from build123d import *

# Parameters (mm, degrees)
MODEL_W                         = 27.94
MODEL_H                         = 50.8
MODEL_R                         = 1.05
MODEL_R_2                       = 5.08
BOSS_EXTRUDE1_DEPTH             = 3.175
F_43_0_089_DIAMETER_HOLE1_D     = 2.2606
F_43_0_089_DIAMETER_HOLE1_DEPTH = 25.4
F_43_0_089_DIAMETER_HOLE1_TIP   = 0.679152758


with BuildPart() as part:
    # Model → Boss-Extrude1 (new body)
    with BuildSketch(Plane.XY):
        with Locations((0, 11.43)):
            Rectangle(MODEL_W, MODEL_H)
        with Locations((-6.92820323, 4.000000001)):
            Circle(MODEL_R, mode=Mode.SUBTRACT)
        with Locations((-6.92820323, -4.000000001)):
            Circle(MODEL_R, mode=Mode.SUBTRACT)
        with Locations((0, -7.999999999)):
            Circle(MODEL_R, mode=Mode.SUBTRACT)
        with Locations((6.92820323, -4.000000001)):
            Circle(MODEL_R, mode=Mode.SUBTRACT)
        with Locations((6.92820323, 4.000000001)):
            Circle(MODEL_R, mode=Mode.SUBTRACT)
        with Locations((0, 7.999999999)):
            Circle(MODEL_R, mode=Mode.SUBTRACT)
        Circle(MODEL_R_2, mode=Mode.SUBTRACT)
    extrude(amount=BOSS_EXTRUDE1_DEPTH)

    # #43 (0.089) Diameter Hole1
    with Locations(Plane.XY.offset(3.175)):
        with Locations((-7.39143302, 7.395974597)):
            Hole(F_43_0_089_DIAMETER_HOLE1_D / 2, depth=F_43_0_089_DIAMETER_HOLE1_DEPTH)
            with Locations((0, 0, -(F_43_0_089_DIAMETER_HOLE1_DEPTH + F_43_0_089_DIAMETER_HOLE1_TIP / 2))):  # 118° drill point
                Cone(0, F_43_0_089_DIAMETER_HOLE1_D / 2, F_43_0_089_DIAMETER_HOLE1_TIP, mode=Mode.SUBTRACT)


solid = part.part
Build history of the part. All positions in model axes, mm. Give positions to 0.01 mm unless a question says otherwise; leave off trailing zeros. Order: outer loops, then holes, each group sorted by start corner. A loop starts at its lowest first (then second) coordinate and runs counter-clockwise, first axis right, second up. Notation, with made-up numbers: M -34,4.5 L -23,4.5 A6 cw -23,15.5 Z; hole C -15.75,43.5 d9. An arc over 180 degrees is marked long. Use one line per item in the form item = value.
Q1. Pull direction X, two halves, no side cores. Call faces 1 (the flat face through (-13.97, 11, 2)), 2 (the flat face through (0, 12, 3.175)), 3 (the cylindrical face through (-5.93, -3.68, 1.57)): released by +X, released by -X, zero draft, split by the parting line, or undercut.
Conclusion:
face_1 = released by -X
face_2 = zero draft
face_3 = undercut
Q2. Slice it at D-D, the plane x = -3. Write the cut outline in (y, z) (3 decimals), and give its area (3 significant figures).
Conclusion:
outline = M -13.97,0 L -4.1,0 L -4.1,3.175 L -13.97,3.175 Z; M 4.1,0 L 36.83,0 L 36.83,3.175 L 4.1,3.175 Z
area = 135 mm2
Q3. Slice it at C-C, the plane y = 8. Write the cut outline in (x, z) (3 decimals).
Conclusion:
outline = M -13.97,0 L -8.347,0 L -8.347,3.175 L -13.97,3.175 Z; M -6.436,0 L -1.05,0 L -1.05,3.175 L -6.436,3.175 Z; M 1.05,0 L 13.97,0 L 13.97,3.175 L 1.05,3.175 Z
Q4. Slice it at A-A, the plane x = 0. Write the cut outline in (y, z) (3 decimals), and give its area (3 significant figures).
Conclusion:
outline = M -13.97,0 L -9.05,0 L -9.05,3.175 L -13.97,3.175 Z; M -6.95,0 L -5.08,0 L -5.08,3.175 L -6.95,3.175 Z; M 5.08,0 L 6.95,0 L 6.95,3.175 L 5.08,3.175 Z; M 9.05,0 L 36.83,0 L 36.83,3.175 L 9.05,3.175 Z
area = 116 mm2
Q5. Wall check: probe 1 along Y at (x, z) = (0, 1.8); probe 2 along Y at (x, z) = (7, 0.6); probe 3 along Y at (x, z) = (7.5, 3). Give the ranges that are in metal, low to high.
Conclusion:
probe_1 = -13.97 to -9.05, -6.95 to -5.08, 5.08 to 6.95, 9.05 to 36.83
probe_2 = -13.97 to -5.05, -2.95 to 2.95, 5.05 to 36.83
probe_3 = -13.97 to -4.88, -3.12 to 3.12, 4.88 to 36.83
Q6. Slice it at B-B, the plane y = 0. Write the cut outline in (x, z) (3 decimals), and give its area (3 significant figures).
Conclusion:
outline = M -13.97,0 L -5.08,0 L -5.08,3.175 L -13.97,3.175 Z; M 5.08,0 L 13.97,0 L 13.97,3.175 L 5.08,3.175 Z
area = 56.5 mm2
